Read the model definition and answer for the solid it produces. Units are mm, in the model's axes. A direction names the side the tool comes from. Coordinates: 2 decimals unless noted, no trailing zeros. Order: outer loops, then holes, each group sorted by start corner. A loop starts at its lowest first (then second) coordinate and runs counter-clockwise, first axis right, second up. Notation, with made-up numbers: (53, 31) -> (86, 31) arc R17 ccw to (86, 44) -> close; hole circle Ø6 at (68.25, 20). An arc over 180 degrees is marked (long way). Use CSV: the item, a comma, the result in double quotes.
Autodesk Inventor part; units mm, degrees
ref_plane "YZ Plane" through (0, 0, 0) normal (1, 0, 0) x (0, 1, 0)
ref_plane "XZ Plane" through (0, 0, 0) normal (0, 1, 0) x (-1, 0, 0)
ref_plane "XY Plane" through (0, 0, 0) normal (0, 0, 1) x (1, 0, 0)
sketch "Sketch1" plane through (0, 0, 0) normal (0, 0, 1) x (1, 0, 0)
  circle A0 centre (0, 0) radius 3.1
  circle A1 centre (0, 0) radius 2.4
  dimension "d0" = 6.2
  dimension "d1" = 4.8
extrude "Extrusion1" add sketch "Sketch1" along normal blind 25.5
sketch "Sketch2" plane through (0, 0, 25.5) normal (0, 0, 1) x (1, 0, 0)
  line L0 (-3.175, 3.175) -> (3.175, 3.175)
  line L1 (3.175, 3.175) -> (3.175, -3.175)
  line L2 (3.175, -3.175) -> (-3.175, -3.175)
  line L3 (-3.175, -3.175) -> (-3.175, 3.175)
  circle A0 centre (0, 0) radius 2.4
  line L4 (-3.175, 3.175) -> (3.175, -3.175) construction
  line L5 (3.175, 3.175) -> (-3.175, -3.175) construction
  dimension "d4" = 6.35
  dimension "d5" = 6.35
extrude "Extrusion2" add sketch "Sketch2" along normal blind 2.5 contours L0 L1 L2 L3 | A0
sketch "Sketch3" plane through (0, 0, 28) normal (0, 0, 1) x (1, 0, 0)
  ellipse E0 centre (0, 0) end of major axis (6.4, 0) minor radius 5.45
  dimension "d8" = 5.45
  dimension "d9" = 6.4
extrude "Extrusion3" add sketch "Sketch3" along normal blind 3
fillet "Fillet1" [suppressed]
fillet "Fillet2" radius 0.5 10 edges at (-3.175, 3.175, 26.75) (3.175, 3.175, 26.75) (0, 3.175, 28) (-3.175, 0, 28) (-3.175, -3.175, 26.75) (0, -3.175, 28) (3.175, -3.175, 26.75) (3.175, 0, 28) (-3.1, 0, 25.5) (-3.1, 0, 0)
thread "Thread1"
properties part number "skaterScrew" material "Stainless Steel"
Item 1: Straight lines are drawn through the part: line 1 along Y through (x, z) = (0, 20); line 2 along Z through (x, y) = (4.75, 3); line 3 along X through (y, z) = (-1, 19.5). For each, find the intervals that lie inside material, in ascending order.
Return value:
line 1,"y = -3.1 to -2.4, 2.4 to 3.1"
line 2,"z = 28 to 31"
line 3,"x = -2.93 to -2.18, 2.18 to 2.93"
Item 2: The mould has two halves that part along Y. Classify faces 4 (the flat face through (0, 0, 25.5)), 5 (the flat face through (0, 3.175, 26)), 6 (the flat face through (0, -3.175, 26)): +Y half, -Y half, draft (parallel to the pull), parting line (faces both ways), or undercut.
Return value:
face 4,"undercut"
face 5,"+Y half"
face 6,"-Y half"
Item 3: Find section A-A, the plane z = 24. Give the vertices of the cut face in (x, y).
Return value:
outline,"circle Ø6.2 at (0, 0); hole circle Ø4.8 at (0, 0)"
Item 4: Each of these flat-tipped pins is pushed along its axis until it touches: P1, Ø3, axis at x = 0, y = 0, coming from the -Z side; P2, Ø0.7, axis at x = 2.5, y = -2, coming from the -Z side; P3, Ø1.5, axis at x = -0.5, z = 16, coming from the +Y side. Where does it stop, or does it pass through?
Return value:
P1,"stops at z = 25.5"
P2,"stops at z = 0.07"
P3,"stops at y = 3.1"
Item 5: A tool of negligible diameter and unlimited length cuts with its end or side. For faces 1 (the flat face through (3.175, 0, 26)), 2 (the flat face through (-2.8, -2.8, 25.5)), 3 (the flat face through (0, 4, 28)), from which of +Z, -Z, +X, -X, +Y, -Y can it reach the whole face along a straight path? Write none if from no direction.
Return value:
face 1,"-Z, +X, +Y, -Y"
face 2,"-Z, -X, -Y"
face 3,"-Z"
